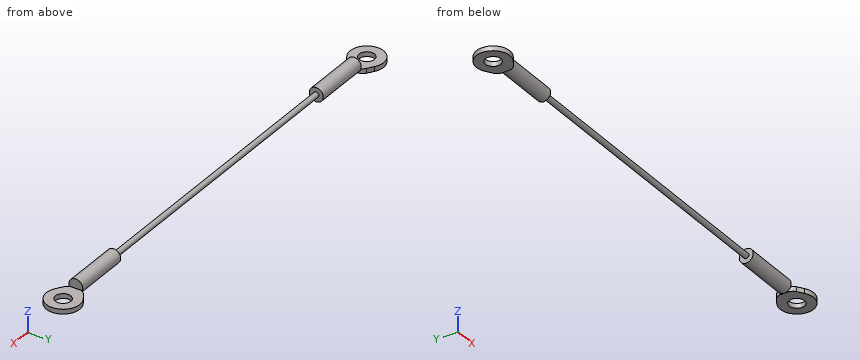
Autodesk Inventor part; units mm, degrees
ref_plane "Work Plane1" through (25.4, 0, 0) normal (1, 0, 0) x (0, 1, 0)
ref_plane "Work Plane2" through (76.2, 0, 0) normal (1, 0, 0) x (0, 1, 0)
ref_plane "XZ Plane" through (0, 0, 0) normal (0, 1, 0) x (-1, 0, 0)
sketch "Sketch1" plane through (0, 0, 0) normal (0, 0, 1) x (1, 0, 0)
  line L0 (0, 7.8788) -> (0, -7.8788)
  line L1 (-8.0232, 0) -> (8.7455, 0)
  circle A0 centre (0, 0) radius 2.5797
  circle A1 centre (0, 0) radius 5.6277
  line L2 (3.1119, 4.689) -> (6.35, 2.54)
  line L3 (6.35, 2.54) -> (6.35, -2.54)
  line L4 (6.35, -2.54) -> (3.1119, -4.689)
  dimension "d0" = 5.1594
  dimension "d1" = 3.048
  dimension "d8" = 6.35
  dimension "d9" = 5.08
extrude "Extrusion1" add sketch "Sketch1" along normal blind 1.5875 contours A1 L1 A0 L0 | L0 A0 L1 A1 | L2 L3 L1 A1 | L1 A0 L0 A1 | L1 A1 L0 A0 | L1 L3 L4 A1
sketch "Sketch2" plane through (0, 0, 0) normal (1, 0, 0) x (0, 1, 0)
  point P0 (0, 0)
ref_plane "Work Plane1" through (25.4, 0, 0) normal (1, 0, 0) x (0, 1, 0)
sketch "Sketch3" plane through (25.4, 0, 0) normal (1, 0, 0) x (0, 1, 0)
  circle A0 centre (0, 2.3495) radius 2.3495
  circle A1 centre (0, 2.3495) radius 0.762
  line L0 (5.6277, 1.5875) -> (-5.6277, 1.5875)
  point P0 (0, 0)
  dimension "d5" = 1.524
extrude "Extrusion2" add sketch "Sketch3" against normal blind 19.05 contours A1 | A0 L0 | L0 A0
fillet "Fillet1" radius 2.54 2 edges at (6.35, 2.54, 0.7937) (6.35, -2.54, 0.7937)
sketch "Sketch4" plane through (25.4, 0, 0) normal (1, 0, 0) x (0, 1, 0)
  circle A0 centre (0, 2.3495) radius 2.3495
  circle A1 centre (0, 2.3495) radius 0.889
  point P0 (0, 0)
  dimension "d11" = 1.778
ref_plane "Work Plane2" through (76.2, 0, 0) normal (1, 0, 0) x (0, 1, 0)
extrude "Extrusion3" add sketch "Sketch4" along normal up to surface (50.8 mm away) contours A1
mirror "Mirror1" about plane through (76.2, 0, 0) normal (1, 0, 0) of "Extrusion3", "Extrusion2", "Fillet1", "Extrusion1"
Part model, mm, in its own coordinate system. Round coordinates to 2 decimals unless told otherwise and drop trailing zeros. Write each loop counter-clockwise with the first axis right and the second up, starting at its lowest first coordinate (ties: lowest second). Pieces come first, ordered by that corner, then holes.
Item 1: Probe L1, parallel to X at y = 0, z = 0.65; L2, parallel to X at y = -1, z = 1.65; L3, parallel to Y at x = 0, z = 0.8. List the from-to ranges inside material, lowest first.
Results:
L1: x = -5.63 to -2.58, 2.58 to 25.4, 127 to 149.82, 154.98 to 158.03
L2: x = 6.35 to 25.4, 127 to 146.05
L3: y = -5.63 to -2.58, 2.58 to 5.63
Item 2: Drop flat-ended pins along their axis: pin 1 Ø2 at (x, y) = (38, 0.5) entering from -Z; pin 2 Ø0.9 at (y, z) = (0, 3) entering from -X; pin 3 Ø1.5 at (x, z) = (61.5, 2) entering from +Y; pin 4 Ø4 at (x, y) = (152.4, 0) entering from -Z. Give the stop position or say it passes through.
Results:
pin 1: stops at z = 1.46
pin 2: stops at x = 6.35
pin 3: stops at y = 0.89
pin 4: passes through
Item 3: Cut at B-B, the plane x = 81. Give the cut face in (y, z).
Results:
outline: circle Ø1.78 at (0, 2.35)
Item 4: Cut at A-A, the plane x = 0. Give the cut face in (y, z), plus the area to 3 significant figures.
Results:
outline: (-5.63, 0) - (-2.58, 0) - (-2.58, 1.59) - (-5.63, 1.59) - close; (2.58, 0) - (5.63, 0) - (5.63, 1.59) - (2.58, 1.59) - close
area: 9.68 mm2
Item 5: Cut at C-C, the plane x = 144.5. Give the cut face in (y, z).
Results:
outline: circle Ø4.7 at (0, 2.35)
